Model file for the job. Use its own axes, mm. Face numbers are marked on the shaded views. A direction names the side the tool comes from. Give positions to 0.01 mm unless a question says otherwise; leave off trailing zeros. Loops run counter-clockwise (first coordinate to the right, second up) from the corner with the lowest first, then second, coordinate; pieces in that order, holes last. Notation, with made-up numbers: M -20,66 L 32,66 A24 cw 32,94 Z; hole C -32.75,-17.5 d9. An arc over 180 degrees is marked long. Use CSV: the item, a comma, the result in double quotes. Start each with the question number.
(1) Tool access for the marked faces 5, 6 and 7: list every direction of +Z, -Z, +X, -X, +Y, -Y with a clear straight run to the whole face (end or side of a thin tool).
(2) Flat gauge pins, fed straight in: P1, Ø12, axis at x = -4, y = -13.5, coming from the +Z side; P2, Ø8, axis at y = -11.5, z = 6.5, coming from the -X side; P3, Ø6, axis at y = -6.5, z = 6.5, coming from the -X side. Where does each tip first touch, or does it go through?
(3) Slice it at D-D on y = -8.5. List the corners of the cut face in (x, z), and give its area (3 significant figures).
(4) Wall check: line 1 along Z through (x, y) = (0.25, -4); line 2 along Z through (x, y) = (-9, 2); line 3 along Y through (x, z) = (-1.75, 9). Give the ranges that are in metal, low to high. Write a range as from..to.
(5) Slice it at B-B on x = 0. List the corners of the cut face in (y, z).
(6) Slice it at A-A on y = 0. List the corners of the cut face in (x, z).
(7) Two-plate mould, pull along Z, no slides. Class the marked faces 1, 2, 3 and 4: pulls with the +Z half, pulls with the -Z half, needs draft (parallel to the pull), parting line crosses it, or undercut.
(8) Slice it at C-C on z = 2. List the corners of the cut face in (x, y), and give its area (3 significant figures).
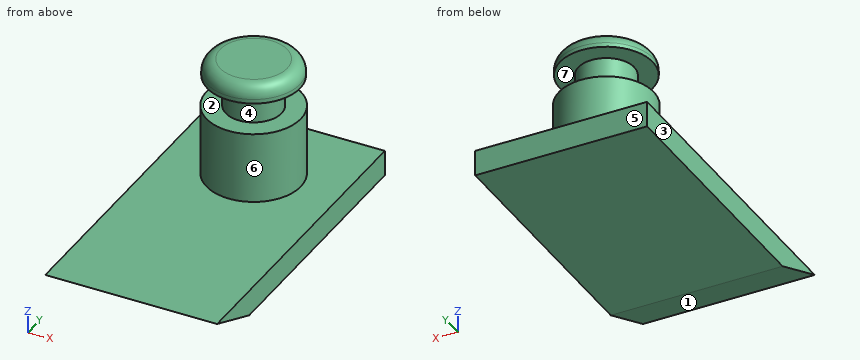
Autodesk Inventor part; units mm, degrees
ref_plane "YZ Plane" through (0, 0, 0) normal (1, 0, 0) x (0, 1, 0)
ref_plane "XZ Plane" through (0, 0, 0) normal (0, 1, 0) x (-1, 0, 0)
ref_plane "XY Plane" through (0, 0, 0) normal (0, 0, 1) x (1, 0, 0)
sketch "Sketch1" plane through (0, 0, 0) normal (0, 0, 1) x (1, 0, 0)
  circle A0 centre (0, 0) radius 5.5
  dimension "d0" = 11
extrude "Extrusion1" add sketch "Sketch1" along normal blind 8.3
sketch "Sketch2" plane through (0, 0, 8.3) normal (0, 0, 1) x (1, 0, 0)
  circle A0 centre (0, 0) radius 3.25
  dimension "d3" = 6.5
extrude "Extrusion2" add sketch "Sketch2" along normal blind 3.7
sketch "Sketch3" plane through (0, 0, 12) normal (0, 0, 1) x (1, 0, 0)
  circle A0 centre (0, 0) radius 5.4
  dimension "d6" = 10.8
extrude "Extrusion3" add sketch "Sketch3" along normal blind 2
fillet "Fillet1" radius 1.5 1 edges at (-5.4, 0, 14)
sketch "Sketch4" plane through (0, 0, 0) normal (0, 0, -1) x (-1, 0, 0)
  line L0 (-10, 10) -> (10, 10)
  line L1 (10, 10) -> (10, -20)
  line L2 (10, -20) -> (-10, -20)
  line L3 (-10, -20) -> (-10, 10)
  point P0 (0, 0)
  dimension "d10" = 20
  dimension "d11" = 30
  dimension "d12" = 10
  dimension "d13" = 10
extrude "Extrusion4" add sketch "Sketch4" along normal blind 3
sketch "Sketch5" plane through (10, -20, 0) normal (1, 0, 0) x (0, 0, -1)
  line L0 (0, 0) -> (0, -6)
  line L1 (0, -6) -> (0, -7.1122)
  line L2 (0, -7.1122) -> (3, 0)
  line L3 (3, 0) -> (0, 0)
  point P0 (0, 20)
  dimension "d16" = 6
extrude "Extrusion5" add sketch "Sketch5" against normal up to surface (20 mm away)
properties part number "vtail_body_piece"
Reply:
1,face 5,"+Z, -Z, +X, -X, +Y"
1,face 6,"+Z"
1,face 7,"none"
2,P1,"stops at z = 0"
2,P2,"passes through"
2,P3,"stops at x = -4.24"
3,outline,"M -10,-3 L 10,-3 L 10,0 L -10,0 Z"
3,area,"60.0 mm^2"
4,line 1,"z = -3..8.3, 12..14"
4,line 2,"z = -3..0"
4,line 3,"y = -2.74..2.74"
5,outline,"M -27.11,0 L -20,-3 L 10,-3 L 10,0 L 5.5,0 L 5.5,8.3 L 3.25,8.3 L 3.25,12 L 5.4,12 L 5.4,12.5 A1.5 ccw 3.9,14 L -3.9,14 A1.5 ccw -5.4,12.5 L -5.4,12 L -3.25,12 L -3.25,8.3 L -5.5,8.3 L -5.5,0 Z"
6,outline,"M -10,-3 L 10,-3 L 10,0 L 5.5,0 L 5.5,8.3 L 3.25,8.3 L 3.25,12 L 5.4,12 L 5.4,12.5 A1.5 ccw 3.9,14 L -3.9,14 A1.5 ccw -5.4,12.5 L -5.4,12 L -3.25,12 L -3.25,8.3 L -5.5,8.3 L -5.5,0 L -10,0 Z"
7,face 1,"pulls with the -Z half"
7,face 2,"undercut"
7,face 3,"needs draft"
7,face 4,"undercut"
8,outline,"C 0,0 d11"
8,area,"95.0 mm^2"
